Autodesk Inventor part; units mm, degrees
ref_plane "Work Plane3" through (0, 0.5, 0) normal (0, 1, 0) x (1, 0, 0)
ref_plane "YZ Plane" through (0, 0, 0) normal (1, 0, 0) x (0, 1, 0)
ref_plane "XZ Plane" through (0, 0, 0) normal (0, 1, 0) x (-1, 0, 0)
sketch "Sketch1" plane through (0, 0, 0) normal (0, 1, 0) x (-1, 0, 0)
  line L0 (21.5102, 17.7267) -> (21.5102, -43.9733)
  line L1 (21.5102, -43.9733) -> (19.1102, -46.7733)
  line L2 (19.1102, -46.7733) -> (-5.4898, -46.7733)
  line L3 (-5.4898, -46.7733) -> (-7.4898, -44.7733)
  line L4 (-7.4898, -44.7733) -> (-7.4898, 9.2267)
  line L5 (-7.4898, 9.2267) -> (5.5102, 22.2267)
  line L6 (5.5102, 22.2267) -> (17.0102, 22.2267)
  line L7 (17.0102, 22.2267) -> (21.5102, 17.7267)
  line L8 (22.0102, 21.7267) -> (22.0102, -46.2733)
  line L9 (22.0102, -46.2733) -> (21.0102, -47.2733)
  line L10 (21.0102, -47.2733) -> (-6.9898, -47.2733)
  line L11 (-6.9898, -47.2733) -> (-7.9898, -46.2733)
  line L12 (-7.9898, -46.2733) -> (-7.9898, 9.7267)
  line L13 (-7.9898, 9.7267) -> (5.0102, 22.7267)
  line L14 (5.0102, 22.7267) -> (21.0102, 22.7267)
  line L15 (21.0102, 22.7267) -> (22.0102, 21.7267)
  point P0 (0, 0)
  point P1 (14.1019, -14.4492)
  dimension "d0" = 69
  dimension "d1" = 29
  dimension "d2" = 2
  dimension "d3" = 2
  dimension "d4" = 2.8
  dimension "d5" = 2.4
  dimension "d6" = 4.5
  dimension "d7" = 4.5
  dimension "d8" = 13
  dimension "d9" = 13
  dimension "d10" = 70
  dimension "d11" = 30
  dimension "d12" = 1
  dimension "d13" = 1
  dimension "d14" = 1
  dimension "d15" = 1
  dimension "d16" = 1
  dimension "d17" = 1
  dimension "d18" = 13
  dimension "d19" = 13
  dimension "d34" = 0.5
  dimension "d35" = 0.5
extrude "Extrusion1" add sketch "Sketch1" along normal blind 3.175 contours L0 L1 L2 L3 L4 L5 L6 L7 | L8 L9 L10 L11 L12 L13 L14 L15
ref_plane "Work Plane3" through (0, 0.5, 0) normal (0, 1, 0) x (1, 0, 0)
sketch "Sketch5" plane through (0, 0.5, 0) normal (0, 1, 0) x (1, 0, 0)
  circle A0 centre (-20.3864, -20.9025) radius 1
  circle A1 centre (-20.8742, 46.0372) radius 0.5
  circle A2 centre (7.0371, 46.2575) radius 0.5
  point P0 (0, 0)
  dimension "d55" = 2
  dimension "d56" = 1
  dimension "d57" = 1
extrude "Extrusion6" cut sketch "Sketch5" along normal blind 3.175 and the other way blind 1.6002
equation "\"d9\" = d8"
equation "\"d19\" = d18"
properties part number "Top"
Design review of the part built by this model. Coordinates are the model's own, in mm. Round coordinates to 2 decimals unless told otherwise and drop trailing zeros. Write each loop counter-clockwise with the first axis right and the second up, starting at its lowest first coordinate (ties: lowest second). Pieces come first, ordered by that corner, then holes.
Item 1: We need section C-C on x = -3.25. Write out the cut boundary in (y, z) (1 decimal), and give its area (3 significant figures).
Item 2: We need section B-B on z = 15.5. Write out the cut boundary in (x, y) (1 decimal).
Item 3: Clearance check with a flat-ended pin moving along its axis: pin 1 Ø1.8 at (x, z) = (-20.39, 20.9) entering from -Y. State where the tip first meets the part, or that it passes through.
Item 4: For probe 1 along Z at (x, y) = (-2, 1.65); probe 2 along Z at (x, y) = (4.25, 1.9), list the stretches that pass through material, from the lowest coordinate up.
Item 5: We need section A-A on y = 2.4. Write out the cut boundary in (x, z), and give its area (3 significant figures).
Returned:
1. outline: (0, -47.3) - (3.2, -47.3) - (3.2, 21) - (0, 21) - close
1. area: 217 mm2
2. outline: (-22, 0) - (2.2, 0) - (2.2, 3.2) - (-22, 3.2) - close
3. pin 1: passes through
4. probe 1: z = -47.27 to 19.72
4. probe 2: z = -47.27 to 13.47
5. outline: (-22.01, -46.27) - (-21.01, -47.27) - (6.99, -47.27) - (7.99, -46.27) - (7.99, 9.73) - (-5.01, 22.73) - (-21.01, 22.73) - (-22.01, 21.73) - close; hole circle Ø2 at (-20.39, 20.9); hole circle Ø1 at (-20.87, -46.04); hole circle Ø1 at (7.04, -46.26)
5. area: 2,010 mm2
